Could you check a few things on this model? Use its own coordinates, in mm. Coordinates: 2 decimals unless noted, no trailing zeros. Loops run counter-clockwise (first coordinate to the right, second up) from the corner with the lowest first, then second, coordinate; pieces in that order, holes last.
from build123d import *

# Parameters (mm, degrees)
ESQUISSE1_W             = 155
ESQUISSE1_H             = 330
BOSS_EXTRU_1_DEPTH      = 3
ENL_V_MAT_EXTRU_1_DEPTH = 10
ESQUISSE3_R             = 2
ENL_V_MAT_EXTRU_2_DEPTH = 10
ESQUISSE4_R             = 1.75
ENL_V_MAT_EXTRU_3_DEPTH = 10


with BuildPart() as part:
    # Esquisse1 → Boss.-Extru.1 (new body)
    with BuildSketch(Plane.XY):
        with Locations((39.953008068, 105.161286668)):
            Rectangle(ESQUISSE1_W, ESQUISSE1_H)
    extrude(amount=BOSS_EXTRU_1_DEPTH)

    # Esquisse2 → Enlèv. mat.-Extru.1 (cut)
    with BuildSketch(Plane.XY.offset(3)):
        Polygon((-27.546991932, -12.838713332), (-27.546991932, 270.161286668), (-37.546991932, 270.161286668), (-37.546991932, -12.838713332), (-37.546991932, -59.838713332), (14.453008068, -59.838713332), (14.453008068, -12.838713332), align=None)
    extrude(amount=-ENL_V_MAT_EXTRU_1_DEPTH, mode=Mode.SUBTRACT)

    # Esquisse3 → Enlèv. mat.-Extru.2 (cut)
    with BuildSketch(Plane.XY.offset(3)):
        with Locations((51.273516144, -52.338713332)):
            Circle(ESQUISSE3_R)
        with Locations((81.273516144, -52.338713332)):
            Circle(ESQUISSE3_R)
        with Locations((-2.546991932, 257.161286668)):
            Circle(ESQUISSE3_R)
        with Locations((35.453008068, 257.161286668)):
            Circle(ESQUISSE3_R)
        with Locations((59.453008068, 257.161286668)):
            Circle(ESQUISSE3_R)
        with Locations((97.453008068, 257.161286668)):
            Circle(ESQUISSE3_R)
    extrude(amount=-ENL_V_MAT_EXTRU_2_DEPTH, mode=Mode.SUBTRACT)

    # Esquisse4 → Enlèv. mat.-Extru.3 (cut)
    with BuildSketch(Plane.XY.offset(3)):
        with Locations((52.953008068, 18.161286668)):
            Circle(ESQUISSE4_R)
        with Locations((52.953008068, 6.161286668)):
            Circle(ESQUISSE4_R)
        with BuildLine():
            Line((56.953008068, 5.161286668), (56.953008068, 19.161286668))
            ThreePointArc((56.953008068, 19.161286668), (57.831687724, 21.282607011), (59.953008068, 22.161286668))
            Line((59.953008068, 22.161286668), (64.953008068, 22.161286668))
            ThreePointArc((64.953008068, 22.161286668), (67.074328411, 21.282607011), (67.953008068, 19.161286668))
            Line((67.953008068, 19.161286668), (67.953008068, 5.161286668))
            ThreePointArc((67.953008068, 5.161286668), (67.074328411, 3.039966324), (64.953008068, 2.161286668))
            Line((64.953008068, 2.161286668), (59.953008068, 2.161286668))
            ThreePointArc((59.953008068, 2.161286668), (57.831687724, 3.039966324), (56.953008068, 5.161286668))
        make_face()
    extrude(amount=-ENL_V_MAT_EXTRU_3_DEPTH, mode=Mode.SUBTRACT)


solid = part.part
1) Imagine slicing it at A-A on z = 2.25. State how many separate pieces and enclosed holes the cut face has, plus the area to 3 significant figures.
2) If I drill on L1, parallel to Y at x = 52.5, z = 0.6; L2, parallel to Y at x = 51, z = 1.6; L3, parallel to X at y = -13, z = 2.5, over which ranges is the centre line in solid material (lowest first)?
3) Will this pin go through, and if not, where does the flat tip stop? pin 1 (0.9 mm diameter, centred on x = -11.5, z = 2, fed in from -Y).
4) Imagine slicing it at C-C on y = -39. List the corners of the cut face in (x, z) for me, plus the area to 3 significant figures.
5) Imagine slicing it at B-B on x = 11. List the corners of the cut face in (y, z) for me, plus the area to 3 significant figures.
Solved:
1. separate pieces: 1
1. enclosed holes: 9
1. area: 45,600 mm2
2. L1: y = -59.84 to -53.92, -50.76 to 4.47, 7.85 to 16.47, 19.85 to 270.16
2. L2: y = -59.84 to -54.32, -50.36 to 270.16
2. L3: x = 14.45 to 117.45
3. pin 1: stops at y = -12.84
4. outline: (14.45, 0) - (117.45, 0) - (117.45, 3) - (14.45, 3) - close
4. area: 309 mm2
5. outline: (-12.84, 0) - (270.16, 0) - (270.16, 3) - (-12.84, 3) - close
5. area: 849 mm2
